The listing builds one solid part. Answer for the finished solid, in the listing's coordinates (mm). Give positions to 0.01 mm unless a question says otherwise; leave off trailing zeros. Use one line per item in the form item = value. Start each with the question number.
1. The part is cut by section A-A (z = -2.25). Give the number of separate pieces and of enclosed holes in the cut face, and give its area (3 significant figures).
2. Straight lines are drawn through the part: line 1 (Z direction, x = 420.5, y = 4.5); line 2 (Z direction, x = 72, y = -5.5); line 3 (Y direction, x = 538, z = -3.2). For each, find the intervals that lie inside material, in ascending order. Write a range as from..to.
3. This flat-tipped pin is pushed along its axis until it touches: pin 1 Ø5 at (x, y) = (63, 0) entering from +Z. Where does it stop, or does it pass through?
from build123d import *
from OCP.BRepFilletAPI import BRepFilletAPI_MakeChamfer

# Parameters (mm, degrees)
BOSS_EXTRUDE1_DEPTH = 650
SKETCH2_R           = 1.75
CUT_EXTRUDE1_DEPTH  = 10
SKETCH3_R           = 3
CUT_EXTRUDE2_DEPTH  = 4
CHAMFER1_SIZE       = 0.5
CHAMFER1_SIZE2      = 1.743707222
FILLET1_R           = 0.5


with BuildPart() as part:
    # Sketch1 → Boss-Extrude1 (new body)
    with BuildSketch(Plane(origin=(0, 0, 0), x_dir=(0, 0, -1), z_dir=(1, 0, 0))):
        Polygon((-0.5, 6), (4, 6), (4, -6), (-0.5, -6), (-0.5, -4.25), (-2.5, -4.25), (-2.5, -6), (-4, -6), (-4, 6), (-2.5, 6), (-2.5, 4.25), (-0.5, 4.25), align=None)
    extrude(amount=BOSS_EXTRUDE1_DEPTH)

    # Sketch2 → Cut-Extrude1 (cut)
    with BuildSketch(Plane.XY.offset(4)):
        with Locations((13, 0)):
            Circle(SKETCH2_R)
        with Locations((38, 0)):
            Circle(SKETCH2_R)
        with Locations((63, 0)):
            Circle(SKETCH2_R)
        with Locations((88, 0)):
            Circle(SKETCH2_R)
        with Locations((113, 0)):
            Circle(SKETCH2_R)
        with Locations((138, 0)):
            Circle(SKETCH2_R)
        with Locations((163, 0)):
            Circle(SKETCH2_R)
        with Locations((188, 0)):
            Circle(SKETCH2_R)
        with Locations((213, 0)):
            Circle(SKETCH2_R)
        with Locations((238, 0)):
            Circle(SKETCH2_R)
        with Locations((263, 0)):
            Circle(SKETCH2_R)
        with Locations((288, 0)):
            Circle(SKETCH2_R)
        with Locations((313, 0)):
            Circle(SKETCH2_R)
        with Locations((338, 0)):
            Circle(SKETCH2_R)
        with Locations((363, 0)):
            Circle(SKETCH2_R)
        with Locations((388, 0)):
            Circle(SKETCH2_R)
        with Locations((413, 0)):
            Circle(SKETCH2_R)
        with Locations((438, 0)):
            Circle(SKETCH2_R)
        with Locations((463, 0)):
            Circle(SKETCH2_R)
        with Locations((488, 0)):
            Circle(SKETCH2_R)
        with Locations((513, 0)):
            Circle(SKETCH2_R)
        with Locations((538, 0)):
            Circle(SKETCH2_R)
        with Locations((563, 0)):
            Circle(SKETCH2_R)
        with Locations((588, 0)):
            Circle(SKETCH2_R)
        with Locations((613, 0)):
            Circle(SKETCH2_R)
        with Locations((638, 0)):
            Circle(SKETCH2_R)
    extrude(amount=-CUT_EXTRUDE1_DEPTH, mode=Mode.SUBTRACT)

    # Sketch3 → Cut-Extrude2 (cut)
    with BuildSketch(Plane.XY.offset(4)):
        with Locations((13, 0)):
            Circle(SKETCH3_R)
        with Locations((38, 0)):
            Circle(SKETCH3_R)
        with Locations((63, 0)):
            Circle(SKETCH3_R)
        with Locations((88, 0)):
            Circle(SKETCH3_R)
        with Locations((113, 0)):
            Circle(SKETCH3_R)
        with Locations((138, 0)):
            Circle(SKETCH3_R)
        with Locations((163, 0)):
            Circle(SKETCH3_R)
        with Locations((188, 0)):
            Circle(SKETCH3_R)
        with Locations((213, 0)):
            Circle(SKETCH3_R)
        with Locations((238, 0)):
            Circle(SKETCH3_R)
        with Locations((263, 0)):
            Circle(SKETCH3_R)
        with Locations((288, 0)):
            Circle(SKETCH3_R)
        with Locations((313, 0)):
            Circle(SKETCH3_R)
        with Locations((338, 0)):
            Circle(SKETCH3_R)
        with Locations((363, 0)):
            Circle(SKETCH3_R)
        with Locations((388, 0)):
            Circle(SKETCH3_R)
        with Locations((413, 0)):
            Circle(SKETCH3_R)
        with Locations((438, 0)):
            Circle(SKETCH3_R)
        with Locations((463, 0)):
            Circle(SKETCH3_R)
        with Locations((488, 0)):
            Circle(SKETCH3_R)
        with Locations((513, 0)):
            Circle(SKETCH3_R)
        with Locations((538, 0)):
            Circle(SKETCH3_R)
        with Locations((563, 0)):
            Circle(SKETCH3_R)
        with Locations((588, 0)):
            Circle(SKETCH3_R)
        with Locations((613, 0)):
            Circle(SKETCH3_R)
        with Locations((638, 0)):
            Circle(SKETCH3_R)
    extrude(amount=-CUT_EXTRUDE2_DEPTH, mode=Mode.SUBTRACT)

    # Chamfer1: one chamfer whose edges measure the first distance from different faces: ONE call of the kernel's chamfer builder (chamfer() names one face for all edges)
    chamfer1_edges_1 = [part.edges().sort_by_distance(p)[0] for p in [
        (325, -4.25, 0.5),
        (325, -4.25, 2.5),
    ]]
    chamfer1_side_1 = [part.faces().sort_by_distance(p)[0] for p in [
        (325, -4.25, 1.5),
    ]]
    chamfer1_edges_2 = [part.edges().sort_by_distance(p)[0] for p in [
        (325, 4.25, 2.5),
        (325, 4.25, 0.5),
    ]]
    chamfer1_side_2 = [part.faces().sort_by_distance(p)[0] for p in [
        (325, 4.25, 1.5),
    ]]
    chamfer1 = BRepFilletAPI_MakeChamfer(part.part.solid().wrapped)
    for e in chamfer1_edges_1:
        chamfer1.Add(CHAMFER1_SIZE, CHAMFER1_SIZE2, e.wrapped, chamfer1_side_1[0].wrapped)  # the first distance lies on this face
    for e in chamfer1_edges_2:
        chamfer1.Add(CHAMFER1_SIZE, CHAMFER1_SIZE2, e.wrapped, chamfer1_side_2[0].wrapped)  # the first distance lies on this face
    add(Compound.cast(chamfer1.Shape()), mode=Mode.REPLACE)

    # Fillet1
    fillet1_edges = [part.edges().sort_by_distance(p)[0] for p in [
        (650, -6, -1.75),
        (650, 0, -4),
        (650, 6, -1.75),
        (650, 6, 3.25),
        (650, 0, 4),
        (650, -6, 3.25),
        (0, -6, 3.25),
        (0, -6, -1.75),
        (0, 0, -4),
        (0, 6, -1.75),
        (0, 6, 3.25),
        (0, 0, 4),
        (325, -4.25, 1),
        (325, -4.25, 2),
        (325, 4.25, 2),
        (325, 4.25, 1),
        (325, -6, 4),
        (325, 6, 4),
        (325, -6, -4),
        (325, 6, -4),
    ]]
    fillet(fillet1_edges, radius=FILLET1_R)


solid = part.part
Derived:
q1.separate_pieces = 1
q1.enclosed_holes = 26
q1.area = 7,550 mm2
q2.line_1 = -4..0.94, 2.06..4
q2.line_2 = -4..0.64, 2.36..4
q2.line_3 = -6..-1.75, 1.75..6
q3.pin_1 = 0
